```python
from build123d import *

# Parameters (mm, degrees)
CORTE_EXTRUS_O1_DEPTH      = 127.242712661
CORTE_EXTRUS_O1_DEPTH_BACK = 127.242712661
ESBO_O2_R                  = 3.5


with BuildPart() as part:
    # Esboço1 → Revolução1 (revolve)
    with BuildSketch(Plane(origin=(0, 0, 0), x_dir=(0, 0, -1), z_dir=(1, 0, 0)), mode=Mode.PRIVATE) as revolu_o1_sk:
        Polygon((0, 123.35), (18, 123.35), (19, 122.35), (19, 115.35), (10, 115.35), (10, -122.35), (9, -123.35), (0, -123.35), align=None)
    revolve(revolu_o1_sk.sketch.rotate(Axis((0, 123.35, 0), (0, -1, 0)), 180), axis=Axis((0, 123.35, 0), (0, -1, 0)))

    # Esboço2 → Corte-extrusão1 (cut, two sides: drawn at the far end of the back side and taken through both)
    with BuildSketch(Plane.XY.offset(-CORTE_EXTRUS_O1_DEPTH_BACK)):
        with Locations((0, -114.85)):
            Circle(ESBO_O2_R)
    extrude(amount=CORTE_EXTRUS_O1_DEPTH + CORTE_EXTRUS_O1_DEPTH_BACK, mode=Mode.SUBTRACT)


solid = part.part
```
The listing builds one solid part. Answer for the finished solid, in the listing's coordinates (mm). Give positions to 0.01 mm unless a question says otherwise; leave off trailing zeros. Order: outer loops, then holes, each group sorted by start corner. A loop starts at its lowest first (then second) coordinate and runs counter-clockwise, first axis right, second up. Notation, with made-up numbers: (32.5, 50) -> (54.5, 50) arc R32 ccw to (54.5, 79) -> close; hole circle Ø1 at (-3, 3). An arc over 180 degrees is marked (long way). Answer as a JSON object with one key per item and string values. Group by question number.
Item 1: Consider L1, parallel to Y at x = 0, z = -4; L2, parallel to Y at x = 8, z = 8.5; L3, parallel to X at y = -114.85, z = 2. Determine where each line is inside the solid, lowest interval first. Write a range as from..to.
Item 2: The part is cut by section D-D on y = 26. Write down the section's boundary in (x, z).
Item 3: The part is cut by section A-A on z = 0. Write down the section's boundary in (x, y).
Item 4: The part is cut by section C-C on y = -114.85. Write down the section's boundary in (x, z), and give its area (3 significant figures).
Item 5: Determine the mould class of faces 1 (the flat face through (0, 123.35, 0)), 2 (the cylindrical face through (18.548, 118.801, -4.119)), 3 (the cylindrical face through (-0.759, -118.267, -0.142)), 4 (the flat face through (0, -123.35, 0)) for opening direction Y: pulls with the +Y half, pulls with the -Y half, needs draft (parallel to the pull), parting line crosses it, or undercut.
Item 6: The part is cut by section B-B on x = 0. Write down the section's boundary in (y, z), and give its area (3 significant figures).
Item 7: Flat-ended cylindrical pins translate along their axes: pin 1 (12 mm diameter, centred on x = -8.5, z = 13.5, fed in from -Y); pin 2 (6 mm diameter, centred on x = 8, y = -49, fed in from +Z); pin 3 (1.5 mm diameter, centred on y = 7, z = 0, fed in from +X); pin 4 (5.5 mm diameter, centred on x = 0, y = -114.85, fed in from -Z). Find the tip coordinate at first contact, or state that the pin passes through.
Result set:
{
 "1": {"L1": "-123.35..-118.35, -111.35..123.35", "L2": "115.35..123.35", "L3": "-9.8..-3.5, 3.5..9.8"},
 "2": {"outline": "circle Ø20 at (0, 0)"},
 "3": {"outline": "(-19, 115.35) -> (-10, 115.35) -> (-10, -122.35) -> (-9, -123.35) -> (9, -123.35) -> (10, -122.35) -> (10, 115.35) -> (19, 115.35) -> (19, 122.35) -> (18, 123.35) -> (-18, 123.35) -> (-19, 122.35) -> close; hole circle Ø7 at (0, -114.85)"},
 "4": {"outline": "(-3.5, -9.37) -> (-3.5, 9.37) arc R10 ccw to start; (3.5, -9.37) arc R10 ccw to (3.5, 9.37) -> close", "area": "177 mm²"},
 "5": {"face 1": "pulls with the +Y half", "face 2": "needs draft", "face 3": "undercut", "face 4": "pulls with the -Y half"},
 "6": {"outline": "(-123.35, -9) -> (-122.35, -10) -> (-118.35, -10) -> (-118.35, 10) -> (-122.35, 10) -> (-123.35, 9) -> close; (-111.35, -10) -> (115.35, -10) -> (115.35, -19) -> (122.35, -19) -> (123.35, -18) -> (123.35, 18) -> (122.35, 19) -> (115.35, 19) -> (115.35, 10) -> (-111.35, 10) -> close", "area": "4,940 mm²"},
 "7": {"pin 1": "y = -122.4", "pin 2": "z = 8.66", "pin 3": "x = 10", "pin 4": "through"}
}
